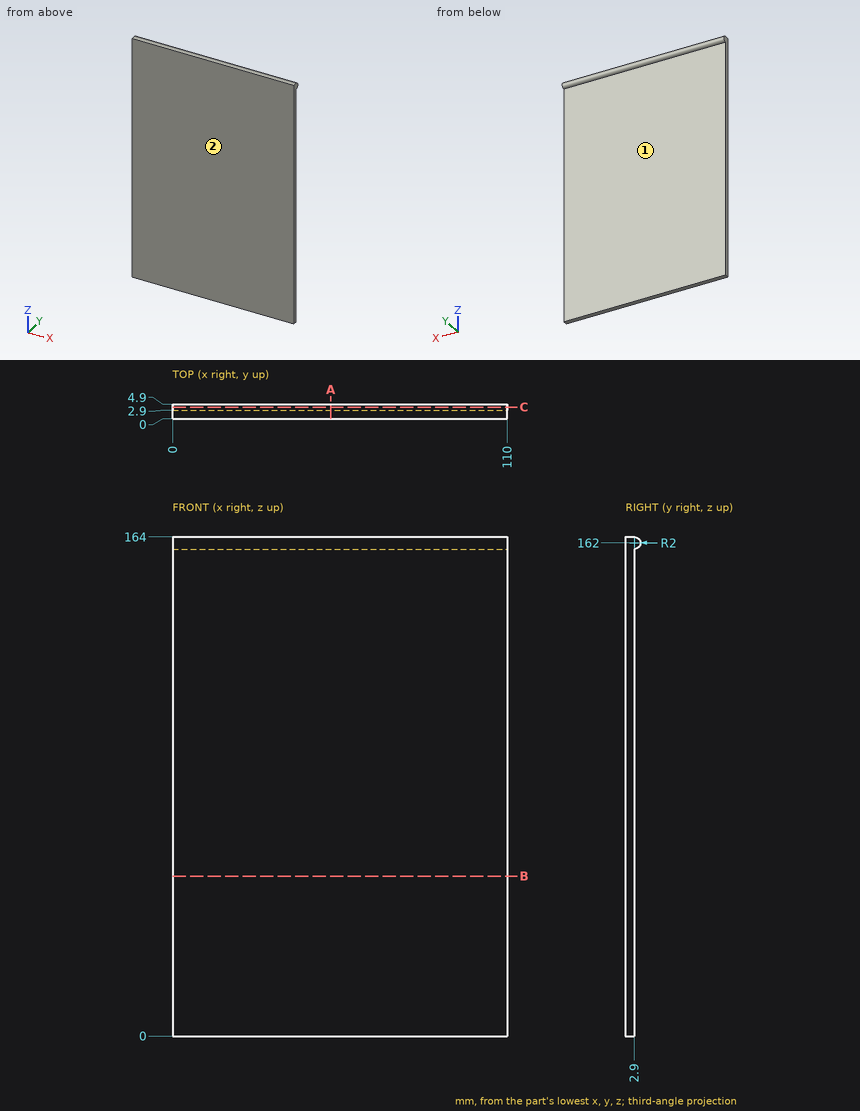
Answer from the drawing. Dimensions are ordinates in mm from the lowest x, y and z of the part. A direction names the side the tool comes from. Give positions to 0.01 mm unless a question says otherwise; leave off trailing zeros. Order: outer loops, then holes, each group sorted by start corner. A loop starts at its lowest first (then second) coordinate and runs counter-clockwise, first axis right, second up. Notation, with made-up numbers: (19.5, 46.5) - (40.5, 46.5) arc R34 cw to (40.5, 83.5) - close; hole circle Ø4 at (-16.5, 38.5). An arc over 180 degrees is marked (long way). One line per item, written item: value. Start each with the question number.
1) Find the intervals of material crossed by L1, parallel to Y at x = 10.5, z = 100; L2, parallel to Z at x = 65.5, y = 3.8; L3, parallel to Z at x = 60.5, y = 3.45, in increasing order.
2) A cutting plane is placed at B-B on z = 52.5. Give the vertices of the cut face in (x, y).
3) Given pin 1 Ø12 at (x, z) = (48.5, 48.5) entering from +Y, flat-ended and moving along its own axis, determine where the tip first touches the part or whether it passes through.
4) A cutting plane is placed at A-A on x = 52. Give the vertices of the cut face in (y, z), then the cut area to 3 significant figures.
5) A tool of negligible diameter and unlimited length cuts with its end or side. For the marked faces 1 and 2, from which of +Z, -Z, +X, -X, +Y, -Y can it reach the whole face along a straight path? Write none if from no direction.
6) A cutting plane is placed at C-C on y = 3.9. Give the vertices of the cut face in (x, z).
Answer sheet:
1. L1: y = 0 to 2.9
1. L2: z = 160.21 to 163.79
1. L3: z = 160.08 to 163.92
2. outline: (0, 0) - (110, 0) - (110, 2.9) - (0, 2.9) - close
3. pin 1: stops at y = 2.9
4. outline: (0, 0) - (2.9, 0) - (2.9, 160) arc R2 ccw to (2.9, 164) - (0, 164) - close
4. area: 482 mm2
5. face 1: -Z, +X, -X, +Y
5. face 2: +Z, -Z, +X, -X, -Y
6. outline: (0, 160.27) - (110, 160.27) - (110, 163.73) - (0, 163.73) - close
